from build123d import *

# Parameters (mm, degrees)
BOSS_EXTRUDE1_DEPTH = 29
SKETCH3_W           = 4.5
SKETCH3_H           = 21
CUT_EXTRUDE1_DEPTH  = 6
SKETCH5_R           = 1.35
BOSS_EXTRUDE2_DEPTH = 4
FILLET1_R           = 1


with BuildPart() as part:
    # Sketch2 → Boss-Extrude1 (new body)
    with BuildSketch(Plane(origin=(0, 0, 0), x_dir=(1, 0, 0), z_dir=(0, 1, 0))):
        with BuildLine():
            Line((0, 10), (0, 20))
            Line((0, 20), (8, 20))
            Line((8, 20), (8, 14.245191882))
            ThreePointArc((8, 14.245191882), (10.672752557, 14.316274399), (13, 13))
            Line((13, 13), (9.464466094, 9.464466094))
            Line((9.464466094, 9.464466094), (2.928932188, 2.928932188))
            ThreePointArc((2.928932188, 2.928932188), (0.761204675, 6.173165676), (0, 10))
        make_face()
    boss_extrude1 = extrude(amount=BOSS_EXTRUDE1_DEPTH)

    # Mirror1: Boss-Extrude1 across plane
    add(boss_extrude1.mirror(Plane(origin=(0, 0, 0), x_dir=(-0.707106781186546, 0, 0.707106781186549), z_dir=(0.707106781186549, 0, 0.707106781186546))))

    # Sketch3 → Cut-Extrude1 (cut)
    with BuildSketch(Plane(origin=(0, 0, -20), x_dir=(-1, 0, 0), z_dir=(0, 0, -1))):
        with Locations((-4, 14.5)):
            Rectangle(SKETCH3_W, SKETCH3_H)
    cut_extrude1 = extrude(amount=-CUT_EXTRUDE1_DEPTH, mode=Mode.SUBTRACT)

    # Mirror2: Cut-Extrude1 across plane
    add(cut_extrude1.mirror(Plane(origin=(0, 0, 0), x_dir=(-0.707106781186546, 0, 0.707106781186549), z_dir=(0.707106781186549, 0, 0.707106781186546))), mode=Mode.SUBTRACT)

    # Sketch5 → Boss-Extrude2 (add)
    with BuildSketch(Plane(origin=(0, 29, 0), x_dir=(1, 0, 0), z_dir=(0, 1, 0))):
        with Locations(Location((9.999139198, 3.962062278, 0), (0, 0, 270))):
            Circle(SKETCH5_R)
        with Locations(Location((3.962062278, 9.999139198, 0), (0, 0, 90))):
            Circle(SKETCH5_R)
    extrude(amount=BOSS_EXTRUDE2_DEPTH)

    # Fillet1
    fillet1_edges = [part.edges().sort_by_distance(p)[0] for p in [
        (9.999139198, 29, -5.312062278),
        (3.962062278, 29, -8.649139198),
    ]]
    fillet(fillet1_edges, radius=FILLET1_R)


solid = part.part
The listing builds one solid part. Answer for the finished solid, in the listing's coordinates (mm). A direction names the side the tool comes from. Give positions to 0.01 mm unless a question says otherwise; leave off trailing zeros. Order: outer loops, then holes, each group sorted by start corner. A loop starts at its lowest first (then second) coordinate and runs counter-clockwise, first axis right, second up. Notation, with made-up numbers: (-31.75, 77.25) - (17.25, 77.25) arc R25 cw to (17.25, 107.25) - close; hole circle Ø3 at (18.5, 55.5). An arc over 180 degrees is marked (long way). Answer as CSV lines item,"result".
Q1. A cutting plane is placed at C-C, the plane y = 25.5. Determine the outline of the cut face in (x, z), and give its area (3 significant figures).
Answer key:
outline,"(0, -20) - (8, -20) - (8, -14.25) arc R5 ccw to (14.25, -8) - (20, -8) - (20, 0) - (10, 0) arc R10 ccw to (0, -10) - close"
area,"271 mm^2"
Q2. A cutting plane is placed at D-D, the plane y = 16. Determine the outline of the cut face in (x, z), and give its area (3 significant figures).
Answer key:
outline,"(0, -20) - (1.75, -20) - (1.75, -14) - (6.25, -14) - (6.25, -20) - (8, -20) - (8, -14.25) arc R5 ccw to (14.25, -8) - (20, -8) - (20, -6.25) - (14, -6.25) - (14, -1.75) - (20, -1.75) - (20, 0) - (10, 0) arc R10 ccw to (0, -10) - close"
area,"217 mm^2"
Q3. Straight lines are drawn through the part: L1, parallel to X at y = 13.5, z = -17.25; L2, parallel to Z at x = 16, y = 11; L3, parallel to Y at x = 3.25, z = -16. For each, find the intervals that lie inside material, in ascending order.
Answer key:
L1,"x = 0 to 1.75, 6.25 to 8"
L2,"z = -8 to -6.25, -1.75 to 0"
L3,"y = 0 to 4, 25 to 29"
Q4. A cutting plane is placed at A-A, the plane z = -16.25. Determine the outline of the cut face in (x, y).
Answer key:
outline,"(0, 0) - (8, 0) - (8, 29) - (0, 29) - close; hole (1.75, 4) - (6.25, 4) - (6.25, 25) - (1.75, 25) - close"
Q5. Determine the mould class of faces 6 (the face through (17, 14, -1.75)), 7 (the face through (4, 33, -10)), 8 (the face through (6.25, 14, -17)), 9 (the face through (7, 14, -20)) for opening direction Y: pulls with the +Y half, pulls with the -Y half, needs draft (parallel to the pull), parting line crosses it, or undercut.
Answer key:
face 6,"undercut"
face 7,"pulls with the +Y half"
face 8,"undercut"
face 9,"needs draft"
Q6. A cutting plane is placed at B-B, the plane x = 18. Determine the outline of the cut face in (y, z), and give its area (4 significant figures).
Answer key:
outline,"(0, -8) - (29, -8) - (29, 0) - (0, 0) - close; hole (4, -6.25) - (25, -6.25) - (25, -1.75) - (4, -1.75) - close"
area,"137.5 mm^2"
Q7. Which of the six approach directions +Z, -Z, +X, -X, +Y, -Y give full straight-line access (tool end or side, diameter ignored) to faces 1 (the face through (15, 14, 0)), 2 (the face through (3.9, 31.48, -8.65)), 3 (the face through (1.75, 14, -17)), 4 (the face through (17, 4, -4)), 5 (the face through (20, 14, -1))?
Answer key:
face 1,"+Z, +X, -X, +Y, -Y"
face 2,"+Y"
face 3,"-Z"
face 4,"+X"
face 5,"+Z, -Z, +X, +Y, -Y"
Q8. Each of these flat-tipped pins is pushed along its axis until it touches: pin 1 Ø1.3 at (y, z) = (19, -3.5) entering from +X; pin 2 Ø6.5 at (x, y) = (18.5, 18.5) entering from -Z; pin 3 Ø5 at (y, z) = (15, -18.5) entering from +X. Where does it stop, or does it pass through?
Answer key:
pin 1,"stops at x = 14"
pin 2,"stops at z = -8"
pin 3,"stops at x = 8"
